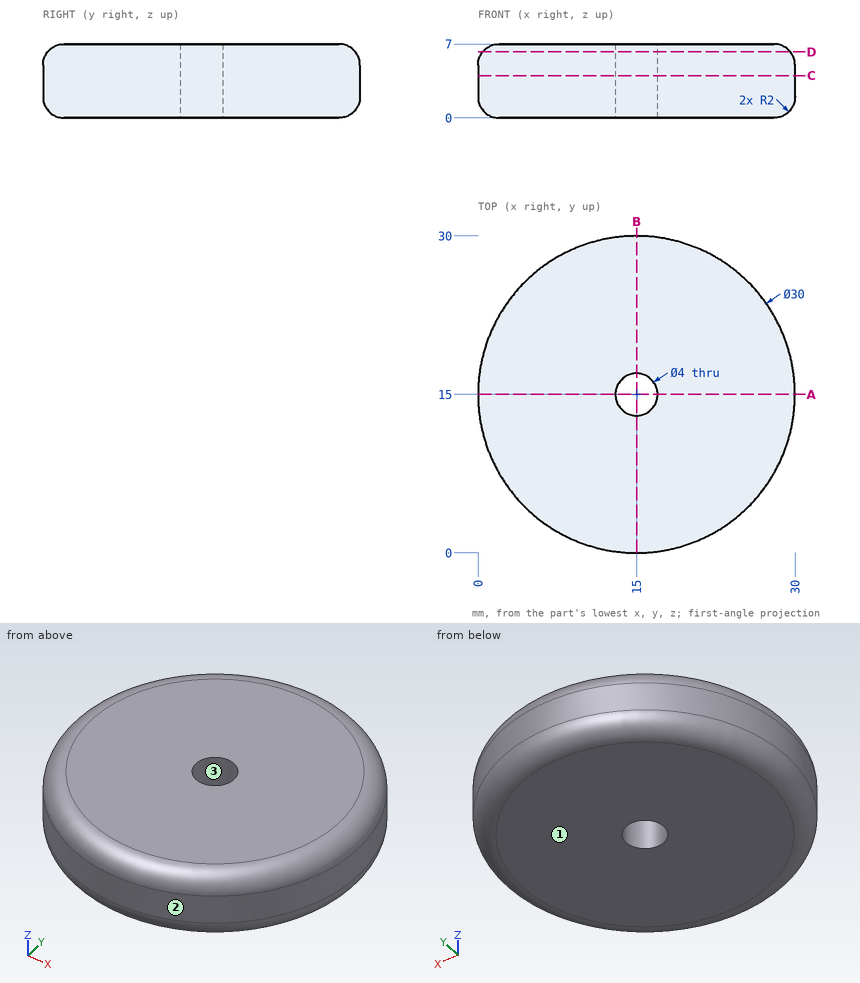
Drawing for the job (mm, zero at the part's lowest x, y, z). Round coordinates to 2 decimals unless told otherwise and drop trailing zeros. Order: outer loops, then holes, each group sorted by start corner. A loop starts at its lowest first (then second) coordinate and runs counter-clockwise, first axis right, second up. Notation, with made-up numbers: (68.5, -28.75) -> (114.5, -28.75) arc R11 ccw to (114.5, -13.75) -> close; hole circle Ø5 at (28.25, 77). An arc over 180 degrees is marked (long way). Put each result on its own line as item: value.
Q1. Pin check, flat tips, straight feed: pin 1 Ø2 at (x, z) = (18.5, 5.5) entering from +Y; pin 2 Ø3 at (x, z) = (12.5, 2) entering from -Y; pin 3 Ø1 at (x, z) = (16, 3) entering from +Y. Stop position of each tip, or through.
From the geometry:
pin 1: stops at y = 29.77
pin 2: stops at y = 0.03
pin 3: stops at y = 29.99
Q2. Band-saw the part on D-D (z = 6.25). Give the cut face in (x, y).
From the geometry:
outline: circle Ø29.12 at (15, 15); hole circle Ø4 at (15, 15)
Q3. Pull direction X, two halves, no side cores. Call the marked faces 1, 2 and 3: pulls with the +X half, pulls with the -X half, needs draft (parallel to the pull), parting line crosses it, or undercut.
From the geometry:
face 1: needs draft
face 2: parting line crosses it
face 3: undercut
Q4. Band-saw the part on C-C (z = 4). Give the cut face in (x, y), and give its area (3 significant figures).
From the geometry:
outline: circle Ø30 at (15, 15); hole circle Ø4 at (15, 15)
area: 694 mm2
Q5. Band-saw the part on A-A (y = 15). Give the cut face in (x, z).
From the geometry:
outline: (0, 2) arc R2 ccw to (2, 0) -> (13, 0) -> (13, 7) -> (2, 7) arc R2 ccw to (0, 5) -> close; (17, 0) -> (28, 0) arc R2 ccw to (30, 2) -> (30, 5) arc R2 ccw to (28, 7) -> (17, 7) -> close
Q6. Wall check: line 1 (Y direction, x = 15, z = 2); line 2 (Y direction, x = 15, z = 1.5); line 3 (X direction, y = 23.5, z = 3). Give the ranges that are in metal, low to high. Write a range as [from, to].
From the geometry:
line 1: y = [0, 13], [17, 30]
line 2: y = [0.06, 13], [17, 29.94]
line 3: x = [2.64, 27.36]
